Model file for the job. Use its own axes, mm. A direction names the side the tool comes from. Coordinates: 2 decimals unless noted, no trailing zeros. Order: outer loops, then holes, each group sorted by start corner. A loop starts at its lowest first (then second) coordinate and runs counter-clockwise, first axis right, second up.
from build123d import *

# Parameters (mm, degrees)
SKETCH1_R           = 62.5
SKETCH1_R_2         = 4
SKETCH1_R_3         = 2.5
BOSS_EXTRUDE1_DEPTH = 5
BOSS_EXTRUDE3_DEPTH = 22
CUT_EXTRUDE1_DEPTH  = 20
CUT_EXTRUDE2_DEPTH  = 11
CUT_EXTRUDE3_START  = -5
SKETCH8_R           = 1
CUT_EXTRUDE3_DEPTH  = 5
SKETCH11_R          = 62.5
SKETCH11_R_2        = 12.5
CUT_EXTRUDE6_DEPTH  = 1


with BuildPart() as part:
    # Sketch1 → Boss-Extrude1 (new body)
    # profile 1 of 10: a face of its own
    with BuildSketch(Plane(origin=(0, 0, 0), x_dir=(1, 0, 0), z_dir=(0, 1, 0))):
        with Locations(Location((0, 0, 0), (0, 0, 270))):
            Circle(SKETCH1_R)
        Polygon((-10.823922003, 0), (-7.653668647, 7.653668647), (0, 10.823922003), (7.653668647, 7.653668647), (10.823922003, 0), (7.653668647, -7.653668647), (0, -10.823922003), (-7.653668647, -7.653668647), align=None, mode=Mode.SUBTRACT)
    # profile 2 of 10: a face of its own
    with BuildSketch(Plane(origin=(0, 0, 0), x_dir=(1, 0, 0), z_dir=(0, 1, 0))):
        Circle(SKETCH1_R_2)
        with Locations(Location((0, 0, 0), (0, 0, 270))):
            Circle(SKETCH1_R_3, mode=Mode.SUBTRACT)
    # profile 3 of 10: a face of its own
    with BuildSketch(Plane(origin=(0, 0, 0), x_dir=(1, 0, 0), z_dir=(0, 1, 0))):
        with BuildLine():
            Line((8.856111893, -4.750713856), (9.621478757, -2.902954791))
            Line((9.621478757, -2.902954791), (3.960853476, -0.558247028))
            ThreePointArc((3.960853476, -0.558247028), (3.69551813, -1.530733729), (3.195486611, -2.406006093))
            Line((3.195486611, -2.406006093), (8.856111893, -4.750713856))
        make_face()
    # profile 4 of 10: a face of its own
    with BuildSketch(Plane(origin=(0, 0, 0), x_dir=(1, 0, 0), z_dir=(0, 1, 0))):
        with BuildLine():
            Line((9.621478757, 2.902954791), (8.856111893, 4.750713856))
            Line((8.856111893, 4.750713856), (3.195486611, 2.406006093))
            ThreePointArc((3.195486611, 2.406006093), (3.69551813, 1.530733729), (3.960853476, 0.558247028))
            Line((3.960853476, 0.558247028), (9.621478757, 2.902954791))
        make_face()
    # profile 5 of 10: a face of its own
    with BuildSketch(Plane(origin=(0, 0, 0), x_dir=(1, 0, 0), z_dir=(0, 1, 0))):
        with BuildLine():
            Line((4.750713856, 8.856111893), (2.902954791, 9.621478757))
            Line((2.902954791, 9.621478757), (0.558247028, 3.960853476))
            ThreePointArc((0.558247028, 3.960853476), (1.530733729, 3.69551813), (2.406006093, 3.195486611))
            Line((2.406006093, 3.195486611), (4.750713856, 8.856111893))
        make_face()
    # profile 6 of 10: a face of its own
    with BuildSketch(Plane(origin=(0, 0, 0), x_dir=(1, 0, 0), z_dir=(0, 1, 0))):
        with BuildLine():
            Line((-0.558247028, 3.960853476), (-2.902954791, 9.621478757))
            Line((-2.902954791, 9.621478757), (-4.750713856, 8.856111893))
            Line((-4.750713856, 8.856111893), (-2.406006093, 3.195486611))
            ThreePointArc((-2.406006093, 3.195486611), (-1.530733729, 3.69551813), (-0.558247028, 3.960853476))
        make_face()
    # profile 7 of 10: a face of its own
    with BuildSketch(Plane(origin=(0, 0, 0), x_dir=(1, 0, 0), z_dir=(0, 1, 0))):
        with BuildLine():
            Line((-3.195486611, 2.406006093), (-8.856111893, 4.750713856))
            Line((-8.856111893, 4.750713856), (-9.621478757, 2.902954791))
            Line((-9.621478757, 2.902954791), (-3.960853476, 0.558247028))
            ThreePointArc((-3.960853476, 0.558247028), (-3.69551813, 1.530733729), (-3.195486611, 2.406006093))
        make_face()
    # profile 8 of 10: a face of its own
    with BuildSketch(Plane(origin=(0, 0, 0), x_dir=(1, 0, 0), z_dir=(0, 1, 0))):
        with BuildLine():
            ThreePointArc((-3.195486611, -2.406006093), (-3.69551813, -1.530733729), (-3.960853476, -0.558247028))
            Line((-3.960853476, -0.558247028), (-9.621478757, -2.902954791))
            Line((-9.621478757, -2.902954791), (-8.856111893, -4.750713856))
            Line((-8.856111893, -4.750713856), (-3.195486611, -2.406006093))
        make_face()
    # profile 9 of 10: a face of its own
    with BuildSketch(Plane(origin=(0, 0, 0), x_dir=(1, 0, 0), z_dir=(0, 1, 0))):
        with BuildLine():
            ThreePointArc((-0.558247028, -3.960853476), (-1.530733729, -3.69551813), (-2.406006093, -3.195486611))
            Line((-2.406006093, -3.195486611), (-4.750713856, -8.856111893))
            Line((-4.750713856, -8.856111893), (-2.902954791, -9.621478757))
            Line((-2.902954791, -9.621478757), (-0.558247028, -3.960853476))
        make_face()
    # profile 10 of 10: a face of its own
    with BuildSketch(Plane(origin=(0, 0, 0), x_dir=(1, 0, 0), z_dir=(0, 1, 0))):
        with BuildLine():
            Line((4.750713856, -8.856111893), (2.406006093, -3.195486611))
            ThreePointArc((2.406006093, -3.195486611), (1.530733729, -3.69551813), (0.558247028, -3.960853476))
            Line((0.558247028, -3.960853476), (2.902954791, -9.621478757))
            Line((2.902954791, -9.621478757), (4.750713856, -8.856111893))
        make_face()
    extrude(amount=BOSS_EXTRUDE1_DEPTH)

    # Sketch3 → Boss-Extrude3 (add)
    with BuildSketch(Plane(origin=(0, 5, 0), x_dir=(1, 0, 0), z_dir=(0, 1, 0))):
        with BuildLine():
            Line((-10.823922003, 0), (-10.823922003, 42.913728942))
            Line((-10.823922003, 42.913728942), (-23.5, 42.913728942))
            Line((-23.5, 42.913728942), (-23.5, 57.913728942))
            ThreePointArc((-23.5, 57.913728942), (0, -62.5), (23.5, 57.913728942))
            Line((23.5, 57.913728942), (23.5, 42.913728942))
            Line((23.5, 42.913728942), (10.823922003, 42.913728942))
            Line((10.823922003, 42.913728942), (10.823922003, 0))
            Line((10.823922003, 0), (7.653668647, -7.653668647))
            Line((7.653668647, -7.653668647), (0, -10.823922003))
            Line((0, -10.823922003), (-7.653668647, -7.653668647))
            Line((-7.653668647, -7.653668647), (-10.823922003, 0))
        make_face()
    extrude(amount=BOSS_EXTRUDE3_DEPTH)

    # Sketch4 → Cut-Extrude1 (cut)
    with BuildSketch(Plane(origin=(0, 0, -42.913728942), x_dir=(-1, 0, 0), z_dir=(0, 0, -1))):
        Polygon((-20.5, 25.25), (-21.366025404, 24.75), (-21.366025404, 23.75), (-20.5, 23.25), (-19.633974596, 23.75), (-19.633974596, 24.75), align=None)
        Polygon((-20.5, 8.75), (-21.366025404, 8.25), (-21.366025404, 7.25), (-20.5, 6.75), (-19.633974596, 7.25), (-19.633974596, 8.25), align=None)
        Polygon((20.5, 8.75), (19.633974596, 8.25), (19.633974596, 7.25), (20.5, 6.75), (21.366025404, 7.25), (21.366025404, 8.25), align=None)
        Polygon((20.5, 25.25), (19.633974596, 24.75), (19.633974596, 23.75), (20.5, 23.25), (21.366025404, 23.75), (21.366025404, 24.75), align=None)
    extrude(amount=-CUT_EXTRUDE1_DEPTH, mode=Mode.SUBTRACT)

    # Sketch7 → Cut-Extrude2 (cut)
    with BuildSketch(Plane(origin=(0, 0, -62.5), x_dir=(-1, 0, 0), z_dir=(0, 0, -1))):
        Polygon((-7.5, 4), (7.5, 4), (7.5, 2), (1.5, 2), (1.5, 0), (-1.5, 0), (-1.5, 2), (-7.5, 2), align=None)
    extrude(amount=-CUT_EXTRUDE2_DEPTH, mode=Mode.SUBTRACT)

    # Sketch8 → Cut-Extrude3 (cut)
    with BuildSketch(Plane.XZ.offset(CUT_EXTRUDE3_START)):
        with Locations(Location((-4, -57, 0), (0, 0, 270))):
            Circle(SKETCH8_R)
        with Locations(Location((4, -57, 0), (0, 0, 270))):
            Circle(SKETCH8_R)
    extrude(amount=CUT_EXTRUDE3_DEPTH, mode=Mode.SUBTRACT)

    # Sketch11 → Cut-Extrude6 (cut)
    with BuildSketch(Plane.XZ):
        with Locations(Location((0, 0, 0), (0, 0, 271.375230752))):
            Circle(SKETCH11_R)
        with Locations(Location((0, 0, 0), (0, 0, 270))):
            Circle(SKETCH11_R_2, mode=Mode.SUBTRACT)
    extrude(amount=-CUT_EXTRUDE6_DEPTH, mode=Mode.SUBTRACT)


solid = part.part
Q1. Cut at A-A, the plane y = 15.5. List the corners of the cut face in (x, z).
Established:
outline: (-23.5, -57.91) - (-23.5, -42.91) - (-10.82, -42.91) - (-10.82, 0) - (-7.65, 7.65) - (0, 10.82) - (7.65, 7.65) - (10.82, 0) - (10.82, -42.91) - (23.5, -42.91) - (23.5, -57.91) arc R62.5 ccw (long way) to start
Q2. Mould opens along Y. For faces 4 (the face through (-23.5, 16, -50)), 5 (the face through (-13, 1, 1)), 6 (the face through (4.5, 2, -55.8)) say: pulls with the +Y half, pulls with the -Y half, needs draft (parallel to the pull), parting line crosses it, or undercut.
Established:
face 4: needs draft
face 5: pulls with the -Y half
face 6: undercut
Q3. Probe line 1 (X direction, y = 4.75, z = -57); line 2 (X direction, y = 1.25, z = -57); line 3 (Y direction, x = 39, z = 44). List the from-to ranges inside material, lowest first.
Established:
line 1: x = -25.64 to -5, -3 to 3, 5 to 25.64
line 2: x = -25.64 to -5, -3 to -1.5, 1.5 to 3, 5 to 25.64
line 3: y = 1 to 27
Q4. Cut at B-B, the plane x = 55. List the corners of the cut face in (y, z), plus the area to 3 significant figures.
Established:
outline: (1, -29.69) - (27, -29.69) - (27, 29.69) - (1, 29.69) - close
area: 1,540 mm2
Q5. Drop flat-ended pins along their axis: P1, Ø0.5, axis at y = 8, z = -30.5, coming from the +X side; P2, Ø12, axis at x = 35, z = -28.5, coming from the -Y side; P3, Ø1.9, axis at x = -21, y = 7.5, coming from the -Z side. Give the stop position or say it passes through.
Established:
P1: stops at x = 54.69
P2: stops at y = 1
P3: stops at z = -42.91
Q6. Which spindle directions (+Z, -Z, +X, -X, +Y, -Y) get a long thin tool onto all of the face, cutting with end or side? Do faces 1 (the face through (1.43, 2.46, -10.23)), 2 (the face through (3.755, 0.493, -11.923)), 3 (the face through (9.261, 13.311, 3.773)). Say none if no direction does.
Established:
face 1: +Y, -Y
face 2: -Y
face 3: +Y
